Part model, mm, in its own coordinate system. A direction names the side the tool comes from. Give positions to 0.01 mm unless a question says otherwise; leave off trailing zeros. Loops run counter-clockwise (first coordinate to the right, second up) from the corner with the lowest first, then second, coordinate; pieces in that order, holes last. Notation, with made-up numbers: M 65.25,44.25 L 109.25,44.25 A33 cw 109.25,83.25 Z; hole C 68,29.25 d6. An arc over 180 degrees is marked long. Answer in a Markdown table with one row per item.
from build123d import *

# Parameters (mm, degrees)
SKETCH_1_W          = 60
SKETCH_1_H          = 90
EXTRUDE_1_DEPTH     = 8
CUT_EXTRUDE_1_REACH = 98.762
SKETCH_3_R          = 2
CUT_EXTRUDE_2_DEPTH = 97.762010118
SKETCH_4_R          = 1.5
CUT_EXTRUDE_3_DEPTH = 76.425459893


with BuildPart() as part:
    # 草图1 → 凸台-拉伸1 (new body)
    with BuildSketch(Plane.XY):
        with Locations((-55.287083442, 0)):
            Rectangle(SKETCH_1_W, SKETCH_1_H)
    extrude(amount=EXTRUDE_1_DEPTH)

    # 草图2 → 切除-拉伸1 (cut, up to next)
    with BuildSketch(Plane.XY.offset(8), mode=Mode.PRIVATE) as cut_extrude_1_sk1:
        Polygon((-81, 17), (-81, 23), (-31, 23), (-31, 17), (-31, -17), (-31, -23), (-81, -23), (-81, -17), align=None)
    cut_extrude_1_tool1 = extrude(cut_extrude_1_sk1.sketch, amount=-CUT_EXTRUDE_1_REACH, mode=Mode.PRIVATE) & part.part
    add(cut_extrude_1_tool1.solids().sort_by_distance((-56, 0, 8))[0], mode=Mode.SUBTRACT)

    # 草图3 → 切除-拉伸2 (cut, through all)
    with BuildSketch(Plane.XY.offset(8)):
        with Locations((-75.287083442, -40)):
            Circle(SKETCH_3_R)
        with Locations((-35.287083442, -40)):
            Circle(SKETCH_3_R)
    cut_extrude_2 = extrude(amount=-CUT_EXTRUDE_2_DEPTH, mode=Mode.SUBTRACT)

    # 镜向1: 切除-拉伸2 across plane
    add(cut_extrude_2.mirror(Plane.ZX), mode=Mode.SUBTRACT)

    # 草图4 → 切除-拉伸3 (cut, through all)
    with BuildSketch(Plane.ZY.offset(85.287083442)):
        with Locations((4, -8.747446088)):
            Circle(SKETCH_4_R)
        with Locations((4, 9.252553912)):
            Circle(SKETCH_4_R)
    extrude(amount=-CUT_EXTRUDE_3_DEPTH, mode=Mode.SUBTRACT)


solid = part.part
(1) Pull direction Z, two halves, no side cores. Call faces 1 (the face through (-29, 1, 8)), 2 (the face through (-29, 1, 0)), 3 (the face through (-83.174, 8.678, 5.386)), 4 (the face through (-35.721, -41.952, 4.056)): +Z half, -Z half, draft (parallel to the pull), parting line (faces both ways), or undercut.
Recorded:
| item | result |
|---|---|
| face 1 | +Z half |
| face 2 | -Z half |
| face 3 | undercut |
| face 4 | draft |
(2) Saw through at D-D (y = 40). Write the cut outline in (x, z), plus the area to 3 significant figures.
Recorded:
| item | result |
|---|---|
| outline | M -85.29,0 L -77.29,0 L -77.29,8 L -85.29,8 Z; M -73.29,0 L -37.29,0 L -37.29,8 L -73.29,8 Z; M -33.29,0 L -25.29,0 L -25.29,8 L -33.29,8 Z |
| area | 416 mm^2 |
(3) Saw through at C-C (x = -63.5). Write the cut outline in (y, z), plus the area to 3 significant figures.
Recorded:
| item | result |
|---|---|
| outline | M -45,0 L -23,0 L -23,8 L -45,8 Z; M 23,0 L 45,0 L 45,8 L 23,8 Z |
| area | 352 mm^2 |
(4) Saw through at A-A (z = 4). Write the cut outline in (x, y), plus the area to 3 significant figures.
Recorded:
| item | result |
|---|---|
| outline | M -85.29,-45 L -25.29,-45 L -25.29,-10.25 L -31,-10.25 L -31,-23 L -81,-23 L -81,-10.25 L -85.29,-10.25 Z; M -85.29,-7.25 L -81,-7.25 L -81,7.75 L -85.29,7.75 Z; M -85.29,10.75 L -81,10.75 L -81,23 L -31,23 L -31,10.75 L -25.29,10.75 L -25.29,45 L -85.29,45 Z; M -31,-7.25 L -25.29,-7.25 L -25.29,7.75 L -31,7.75 Z; hole C -75.29,-40 d4; hole C -75.29,40 d4; hole C -35.29,-40 d4; hole C -35.29,40 d4 |
| area | 2,990 mm^2 |
(5) Pin check, flat tip, straight feed: pin 1 Ø2.5 at (y, z) = (-8.75, 4) entering from +X. Stop position of the tip, or through.
Recorded:
| item | result |
|---|---|
| pin 1 | passes through |
(6) Drill centre lines: line 1 along Y through (x, z) = (-47.5, 1); line 2 along X through (y, z) = (5, 7); line 3 along Y through (x, z) = (-26.65, 4). Where is each one in solid material? Low to high.
Recorded:
| item | result |
|---|---|
| line 1 | y = -45 to -23, 23 to 45 |
| line 2 | x = -85.29 to -81, -31 to -25.29 |
| line 3 | y = -45 to -10.25, -7.25 to 7.75, 10.75 to 45 |
(7) Saw through at B-B (y = 5). Write the cut outline in (x, z), plus the area to 3 significant figures.
Recorded:
| item | result |
|---|---|
| outline | M -85.29,0 L -81,0 L -81,8 L -85.29,8 Z; M -31,0 L -25.29,0 L -25.29,8 L -31,8 Z |
| area | 80.0 mm^2 |
(8) Which spindle directions (+Z, -Z, +X, -X, +Y, -Y) get a long thin tool onto all of the face, cutting with end or side? Do faces 5 (the face through (-56, -23, 4)), 6 (the face through (-56, -45, 4)). Say none if no direction does.
Recorded:
| item | result |
|---|---|
| face 5 | +Z, -Z |
| face 6 | +Z, -Z, +X, -X, -Y |
